Input: part model. Units: mm. Frame: model coordinates. A direction names the side the tool comes from. Round coordinates to 2 decimals unless told otherwise and drop trailing zeros. Write each loop counter-clockwise with the first axis right and the second up, starting at its lowest first coordinate (ties: lowest second). Pieces come first, ordered by that corner, then holes. Notation, with made-up numbers: (78, 77) -> (86, 77) arc R17 ccw to (86, 99) -> close; hole circle Ø8 at (85, -20). An arc over 180 degrees is marked (long way). Use CSV: the item, a comma, the result in double quotes.
```python
from build123d import *

# Parameters (mm, degrees)
CUT_EXTRUDE2_START                              = 9.275318
CUT_EXTRUDE2_OUTLINE_R                          = 47.625
CUT_EXTRUDE2_DEPTH                              = 8.504682
CBORE_FOR_10_SOCKET_HEAD_CAP_SCREW1_D           = 4.9784
CBORE_FOR_10_SOCKET_HEAD_CAP_SCREW1_CBORE_D     = 9.525
CBORE_FOR_10_SOCKET_HEAD_CAP_SCREW1_CBORE_DEPTH = 4.826
F_10_CLEARANCE_HOLE1_D                          = 5.1054
CIRPATTERN1_COUNT                               = 8
CLEARANCING_START                               = -8.504682
SKETCH25_R                                      = 66.675
CLEARANCING_DEPTH                               = 8.504682


# Read off the part's stored shape, not the designer's step: Cut-Extrude2
with BuildPart() as part:
    # Sketch24 → Revolve1 (revolve)
    with BuildSketch(Plane(origin=(0, 0, 0), x_dir=(1, 0, 0), z_dir=(0, 1, 0))):
        Polygon((-15.875, -33.405318), (-15.875, -17.78), (-34.29, -17.78), (-34.29, -9.275318), (-47.625, -9.275318), (-47.625, -17.78), (-46.0248, -17.78), (-46.0248, -20.9169), (-50.8, -20.9169), (-50.8, -17.78), (-66.675, -17.78), (-66.675, -33.405318), align=None)
    revolve(axis=Axis((0, 0, 0), (0, 0, 1)))

    # Cut-Extrude2 outline → Cut-Extrude2 (cut)
    with BuildSketch(Plane.XY.offset(CUT_EXTRUDE2_START)):
        Circle(CUT_EXTRUDE2_OUTLINE_R)
        with BuildLine():
            add(Edge.make_bspline(
                [(34.641574854, 11.209813305), (34.492866613, 11.743162162), (34.153943811, 12.859819093), (33.555538624, 14.537761538), (32.849887572, 16.240636382), (32.057893687, 17.909346365), (31.181197352, 19.53951152), (30.221662701, 21.126830276), (29.181373626, 22.667090912), (28.062629225, 24.156182809), (26.867938753, 25.590107465), (25.60001603, 26.964989265), (24.261773335, 28.277085961), (22.856314773, 29.522798851), (21.386929147, 30.698682629), (19.85708232, 31.801454876), (18.270409111, 32.828005175), (16.630704717, 33.775403815), (14.941915703, 34.640910073), (13.208130556, 35.421980041), (11.43356985, 36.116273987), (9.622576022, 36.721663214), (7.779602801, 37.236236415), (5.909204301, 37.658305492), (4.016023818, 37.986410831), (2.104782347, 38.219326014), (0.180266852, 38.356061949), (-1.75268168, 38.395870413), (-3.689180377, 38.338246992), (-5.624316777, 38.182933409), (-7.553161251, 37.929919231), (-9.470779522, 37.579442948), (-11.37224525, 37.131992419), (-13.252652651, 36.588304682), (-15.107129112, 35.949365124), (-16.930847778, 35.216406011), (-18.719040078, 34.390904381), (-20.467008144, 33.474579298), (-22.170137115, 32.469388481), (-23.823907266, 31.377524301), (-25.42390596, 30.201409162), (-26.965839357, 28.943690275), (-28.445543888, 27.607233836), (-29.858997424, 26.195118613), (-31.202330147, 24.710628968), (-32.471835063, 23.157247319), (-33.663978152, 21.538646066), (-34.775408104, 19.858679), (-35.802965645, 18.121372202), (-36.743692396, 16.330914471), (-37.594839261, 14.491647299), (-38.353874308, 12.608054401), (-39.018490139, 10.68475085), (-39.586610697, 8.726471825), (-40.056397525, 6.738061006), (-40.426255434, 4.724458642), (-40.694837576, 2.690689328), (-40.861049894, 0.641849508), (-40.924054953, -1.416905249), (-40.883275123, -3.480373184), (-40.738395114, -5.543319447), (-40.489363842, -7.600489337), (-40.13639564, -9.646621653), (-39.679970776, -11.676462103), (-39.120835312, -13.684776759), (-38.460000265, -15.666365517), (-37.698740094, -17.61607551), (-36.838590511, -19.528814477), (-35.881345602, -21.399564006), (-34.829054288, -23.223392663), (-33.684016107, -24.995468936), (-32.44877635, -26.711073982), (-31.126120537, -28.365614138), (-29.719068263, -29.954633155), (-28.230866416, -31.473824138), (-26.664981791, -32.919041144), (-25.025093105, -34.286310417), (-23.315082441, -35.571841228), (-21.53902614, -36.772036288), (-19.701185153, -37.883501708), (-17.805994889, -38.903056478), (-15.85805457, -39.827741435), (-13.862116128, -40.654827709), (-11.823072667, -41.381824596), (-9.745946518, -42.006486871), (-7.635876912, -42.526821485), (-5.498107312, -42.941093656), (-3.337972426, -43.247832311), (-1.160884928, -43.445834888), (1.027678058, -43.534171454), (3.222188708, -43.512188152), (5.417082419, -43.379509955), (7.606771886, -43.136042707), (9.785661288, -42.781974466), (11.948160555, -42.317776118), (14.08869967, -41.74420128), (16.201742982, -41.062285471), (18.281803484, -40.273344558), (20.323457017, -39.378972487), (22.321356376, -38.381038284), (24.27024527, -37.281682345), (26.164972102, -36.083312015), (28.000503535, -34.788596469), (29.77193781, -33.400460899), (31.474517775, -31.92208003), (33.103643596, -30.356870964), (34.654885111, -28.708485383), (36.123993806, -26.980801118), (37.506914359, -25.17791311), (38.799795742, -23.304123775), (39.999001844, -21.363932809), (41.101121576, -19.362026441), (42.102978449, -17.303266175), (43.001639577, -15.192677038), (43.794424103, -13.035435358), (44.478911001, -10.836856121), (45.052946246, -8.602379918), (45.514649334, -6.337559517), (45.847889349, -4.143701635), (46.017592475, -2.510533136), (46.090246085, -1.546597167), (46.115686798, -1.160407225), (46.132959236, -0.870548295), (46.148375241, -0.580516781), (46.162099639, -0.290330355), (46.169705769, -0.096784384), (46.173509282, 0)],
                knots=[0.044023807, 0.044023807, 0.044023807, 0.044023807, 0.050477114, 0.057621232, 0.06478017, 0.071953969, 0.079142669, 0.086346306, 0.093564916, 0.100798534, 0.108047194, 0.115310927, 0.122589766, 0.12988374, 0.13719288, 0.144517215, 0.151856774, 0.159211583, 0.16658167, 0.173967063, 0.181367786, 0.188783866, 0.196215328, 0.203662198, 0.211124498, 0.218602253, 0.226095488, 0.233604225, 0.241128486, 0.248668296, 0.256223676, 0.263794648, 0.271381234, 0.278983456, 0.286601335, 0.294234891, 0.301884146, 0.309549121, 0.317229835, 0.324926308, 0.332638561, 0.340366614, 0.348110485, 0.355870195, 0.363645762, 0.371437205, 0.379244543, 0.387067795, 0.39490698, 0.402762115, 0.410633219, 0.41852031, 0.426423405, 0.434342523, 0.442277682, 0.450228898, 0.458196189, 0.466179572, 0.474179065, 0.482194684, 0.490226447, 0.498274369, 0.506338468, 0.514418761, 0.522515263, 0.530627991, 0.538756962, 0.546902191, 0.555063694, 0.563241488, 0.571435588, 0.57964601, 0.58787277, 0.596115883, 0.604375364, 0.61265123, 0.620943495, 0.629252175, 0.637577285, 0.64591884, 0.654276855, 0.662651345, 0.671042324, 0.679449808, 0.687873812, 0.696314349, 0.704771435, 0.713245083, 0.721735309, 0.730242127, 0.738765551, 0.747305595, 0.755862273, 0.7644356, 0.77302559, 0.781632256, 0.790255613, 0.798895674, 0.807552454, 0.816225965, 0.824916222, 0.833623239, 0.842347028, 0.851087604, 0.859844979, 0.868619169, 0.877410184, 0.88621804, 0.895042749, 0.903884325, 0.912742781, 0.921618129, 0.930510383, 0.939419557, 0.948345662, 0.957288712, 0.96624872, 0.975225699, 0.984219661, 0.99210332, 0.994358185, 0.995486016, 0.996614114, 0.997742477, 0.998871105, 1, 1, 1, 1], degree=3))
            ThreePointArc((34.641574854, 11.209813305), (36.735471945, 8.002059693), (40.293337039, 6.582311745))
            ThreePointArc((40.293337039, 6.582311745), (44.564000123, 4.479799319), (46.173509282, 0))
        make_face(mode=Mode.SUBTRACT)
    extrude(amount=CUT_EXTRUDE2_DEPTH, mode=Mode.SUBTRACT)

    # CBORE for #10 Socket Head Cap Screw1 (through all)
    with Locations(Plane(origin=(19.083044257, -19.083044257, 17.78), x_dir=(-1, 0, 0), z_dir=(0, 0, -1))):
        with Locations((0, 0), (0, 38.166088514), (38.166088514, 38.166088514), (38.166088514, 0)):
            CounterBoreHole(CBORE_FOR_10_SOCKET_HEAD_CAP_SCREW1_D / 2, CBORE_FOR_10_SOCKET_HEAD_CAP_SCREW1_CBORE_D / 2, CBORE_FOR_10_SOCKET_HEAD_CAP_SCREW1_CBORE_DEPTH)

    # #10 Clearance Hole1 (through all)
    with Locations(Plane(origin=(55.733032799, -23.085378057, 17.78), x_dir=(-1, 0, 0), z_dir=(0, 0, -1))):
        with Locations((0, 0)):
            f_10_clearance_hole1 = Hole(F_10_CLEARANCE_HOLE1_D / 2)

    # CirPattern1: #10 Clearance Hole1 ×8 about axis
    cirpattern1_axis = Axis((0, 0, 0), (0, 0, 1))
    for i in range(1, CIRPATTERN1_COUNT):
        add(f_10_clearance_hole1.rotate(cirpattern1_axis, i * 360 / CIRPATTERN1_COUNT), mode=Mode.SUBTRACT)

    # Sketch25 → Clearancing (cut)
    with BuildSketch(Plane(origin=(0, 0, 9.275318), x_dir=(-1, 0, 0), z_dir=(0, 0, -1)).offset(CLEARANCING_START)):
        Circle(SKETCH25_R)
        with BuildLine():
            ThreePointArc((-40.256142642, 6.075675212), (-44.185152679, 4.14136378), (-45.665901105, 0.019948406))
            add(Edge.make_bspline(
                [(-45.665901105, 0.019948406), (-45.640843252, -0.617675003), (-45.604829255, -1.253010819), (-45.504351835, -2.517742345), (-45.441052831, -3.147381178), (-45.212432947, -5.028212524), (-45.008450664, -6.271332714), (-44.242989524, -9.968640212), (-43.52913227, -12.391011617), (-42.138045746, -15.957691436), (-41.626364682, -17.120474764), (-40.512680652, -19.388257745), (-39.910207789, -20.494442857), (-37.96707369, -23.730593733), (-36.49174462, -25.778791172), (-34.411771475, -28.195856513), (-33.985279842, -28.670377793), (-33.116423575, -29.596422364), (-32.673332521, -30.04879752), (-31.318399621, -31.37438599), (-30.380949523, -32.216125582), (-27.46704593, -34.616530673), (-25.389841573, -36.05136872), (-22.062172671, -37.943237182), (-20.930130825, -38.522778109), (-18.633091111, -39.57639236), (-17.46623561, -40.051525518), (-13.91112995, -41.323221397), (-11.468273082, -41.967409438), (-6.43242256, -42.826573909), (-3.914744792, -43.028776038), (-0.138586, -43.003300652), (1.120073594, -42.939681088), (3.007971483, -42.760186242), (3.637255506, -42.686322311), (4.895792474, -42.510042802), (5.526571063, -42.407330429), (8.660443645, -41.824544462), (11.090372365, -41.142352886), (14.623012975, -39.804920602), (15.781736724, -39.306432263), (17.491004632, -38.478051741), (18.055949728, -38.188461399), (19.176029707, -37.581826274), (19.731660414, -37.26438738), (22.456662681, -35.624532778), (24.490489311, -34.13384221), (27.326701243, -31.635387766), (28.236132982, -30.758567046), (29.981154487, -28.914599378), (30.819228008, -27.943481359), (33.171025404, -24.950670888), (34.539973674, -22.835332473), (36.297963516, -19.483904717), (36.83442316, -18.336845345), (37.562280382, -16.569855108), (37.792222154, -15.972450916), (38.221480922, -14.774667607), (38.42145983, -14.172789371), (39.349182921, -11.148685634), (39.862263674, -8.682699789), (40.215714934, -5.541527517), (40.271892159, -4.9103345), (40.354705457, -3.641926337), (40.381354461, -3.003087554), (40.415744918, -1.089891477), (40.378321818, 0.17699807), (40.089998698, 3.952653081), (39.66460968, 6.436627246), (38.66814911, 10.111670481), (38.273517277, 11.333002184), (37.378111134, 13.708459229), (36.876425473, 14.867850039), (35.212263321, 18.262501529), (33.892198877, 20.41503772), (31.966087362, 22.960807794), (31.568415192, 23.460588842), (30.753517199, 24.435348736), (30.335543042, 24.911319081), (29.050471233, 26.305463264), (27.254106693, 28.07441755), (25.292803648, 29.664573356), (23.7585556, 30.788602731), (23.23657543, 31.151827317), (22.171009443, 31.854855296), (21.628884127, 32.193593191), (18.893658644, 33.810617118), (16.607565234, 34.874431278), (13.033225917, 36.129365373), (11.817410682, 36.490482396), (9.955700277, 36.942999941), (9.331375211, 37.078252299), (8.083229873, 37.316282707), (7.458193096, 37.419364645), (4.328251999, 37.856154552), (1.809219852, 37.956379859), (-1.992431203, 37.724910244), (-3.268993537, 37.582194436), (-5.774771117, 37.172490518), (-8.244673009, 36.63892044), (-10.644023937, 35.861762645), (-12.416713296, 35.186281009), (-13.003131207, 34.945657629), (-14.166839857, 34.432897949), (-14.74571793, 34.15994609), (-17.595998473, 32.724883965), (-19.722308373, 31.363177043), (-22.686779283, 29.00829021), (-23.637145616, 28.170868672), (-25.003992637, 26.833248229), (-25.450247046, 26.373128306), (-26.31251867, 25.436365373), (-26.729880148, 24.958475365), (-28.748893153, 22.522226272), (-30.149346389, 20.424978266), (-31.921880839, 17.052584644), (-32.458700819, 15.886348957), (-33.400814883, 13.514922144), (-33.808577866, 12.305934879), (-34.152239482, 11.073376896)],
                knots=[0, 0, 0, 0, 0.0078125, 0.0078125, 0.015625, 0.015625, 0.03125, 0.03125, 0.0625, 0.0625, 0.078125, 0.078125, 0.09375, 0.09375, 0.125, 0.125, 0.1328125, 0.1328125, 0.140625, 0.140625, 0.15625, 0.15625, 0.1875, 0.1875, 0.203125, 0.203125, 0.21875, 0.21875, 0.25, 0.25, 0.28125, 0.28125, 0.296875, 0.296875, 0.3046875, 0.3046875, 0.3125, 0.3125, 0.34375, 0.34375, 0.359375, 0.359375, 0.3671875, 0.3671875, 0.375, 0.375, 0.40625, 0.40625, 0.421875, 0.421875, 0.4375, 0.4375, 0.46875, 0.46875, 0.484375, 0.484375, 0.4921875, 0.4921875, 0.5, 0.5, 0.53125, 0.53125, 0.5390625, 0.5390625, 0.546875, 0.546875, 0.5625, 0.5625, 0.59375, 0.59375, 0.609375, 0.609375, 0.625, 0.625, 0.65625, 0.65625, 0.6640625, 0.6640625, 0.671875, 0.671875, 0.6875, 0.703125, 0.703125, 0.7109375, 0.7109375, 0.71875, 0.71875, 0.75, 0.75, 0.765625, 0.765625, 0.7734375, 0.7734375, 0.78125, 0.78125, 0.8125, 0.8125, 0.828125, 0.828125, 0.84375, 0.859375, 0.859375, 0.8671875, 0.8671875, 0.875, 0.875, 0.90625, 0.90625, 0.921875, 0.921875, 0.9296875, 0.9296875, 0.9375, 0.9375, 0.96875, 0.96875, 0.984375, 0.984375, 1, 1, 1, 1], degree=3))
            ThreePointArc((-34.152239482, 11.073376896), (-36.41364834, 7.609002996), (-40.256142642, 6.075675212))
        make_face(mode=Mode.SUBTRACT)
    extrude(amount=CLEARANCING_DEPTH, mode=Mode.SUBTRACT)


solid = part.part
```
Item 1: Line query: line 1 (Y direction, x = 0, z = 19) (3 decimals); line 2 (Y direction, x = 57.5, z = 23.25); line 3 (X direction, y = -54, z = 25.5). Output: solid intervals per line, ascending.
Worked answers:
line 1,"y = -66.675 to -50.8, -46.025 to -15.875, 15.875 to 46.025, 50.8 to 66.675"
line 2,"y = -33.75 to -24.93, -21.24 to 21.24, 24.93 to 33.75"
line 3,"x = -39.11 to -24.96, -21.21 to 21.21, 24.96 to 39.11"
Item 2: Set-up query: faces 1 (the face through (36.368, 7.646, 13.587)), 2 (the face through (-19.623, 16.653, 28.081)), 3 (the face through (20.115, 14.434, 20.159)). Return all of +Z, -Z, +X, -X, +Y, -Y with unobstructed straight access to the full face (end or side cutting, diameter ignored); none if empty.
Worked answers:
face 1,"-Z, +X, +Y"
face 2,"+Z, -Z"
face 3,"-Z"
Item 3: Pull-direction query (X, two-part tool) for faces 4 (the face through (34, 39, 17.78)), 5 (the face through (17, -21, 22.606)), 6 (the face through (-63.596, -20.027, 25.702)); classes: +X half, -X half, draft (parallel to the pull), parting line (faces both ways), or undercut.
Worked answers:
face 4,"draft"
face 5,"undercut"
face 6,"parting line"
Item 4: First-contact query: pin 1 Ø4 at (x, y) = (55.73, -23.09) entering from +Z; pin 2 Ø5.5 at (x, y) = (-19.08, 19.08) entering from -Z; pin 3 Ø2 at (x, z) = (40.5, 19) entering from -Y; pin 4 Ø7.5 at (x, y) = (18, -19.5) entering from -Z. Flat tips, straight axial feed; report the tip coordinate or a pass-through.
Worked answers:
pin 1,"passes through"
pin 2,"stops at z = 22.61"
pin 3,"stops at y = -53.72"
pin 4,"stops at z = 17.78"
Item 5: Section query A-A on y = -49. Return the cut outline in (x, z), plus the area to 3 significant figures.
Worked answers:
outline,"(-45.22, 17.78) -> (-13.4, 17.78) -> (-13.4, 20.92) -> (13.4, 20.92) -> (13.4, 17.78) -> (45.22, 17.78) -> (45.22, 33.41) -> (-45.22, 33.41) -> close"
area,"1,330 mm²"
